Autodesk Fusion 360 part; units mm, degrees
sketch "Sketch1" plane through (0, 0, 0) normal (0, 1, 0) x (1, 0, 0)
  arc A0 (-2, -13.1375) -> (2, -13.1375) centre (0, -11.25) ccw
  line L0 (-2, -13.1375) -> (-2, -9.3625)
  arc A1 (2, -9.3625) -> (-2, -9.3625) centre (0, -11.25) ccw
  line L1 (2, -9.3625) -> (2, -13.1375)
  line L2 (-2.5, -13.3267) -> (-2.5, -9.1733)
  arc A2 (2.5, -9.1733) -> (-2.5, -9.1733) centre (0, -11.25) ccw
  line L3 (2.5, -9.1733) -> (2.5, -13.3267)
  arc A3 (-2.5, -13.3267) -> (2.5, -13.3267) centre (0, -11.25) ccw
  arc A4 (-6, -14.3423) -> (6, -14.3423) centre (0, -11.25) ccw
  line L4 (6, -8.1577) -> (6, -14.3423)
  arc A5 (6, -8.1577) -> (-6, -8.1577) centre (0, -11.25) ccw
  line L5 (-6, -14.3423) -> (-6, -8.1577)
  circle A6 centre (10, -11.25) radius 2.5
  line L6 (2.5219, -17.5112) -> (11.06, -13.5142)
  line L7 (3.1933, -5.3031) -> (11.06, -8.9858)
  line L8 (1.5, -9.5729) -> (1.5, -12.9271)
  arc A7 (-1.5, -12.9271) -> (1.5, -12.9271) centre (0, -11.25) ccw
  line L9 (-1.5, -12.9271) -> (-1.5, -9.5729)
  arc A8 (1.5, -9.5729) -> (-1.5, -9.5729) centre (0, -11.25) ccw
  circle A9 centre (0, -11.25) radius 6.75
  dimension "d1" = 0.5
  dimension "d2" = -4
  dimension "d3" = 5
  dimension "d4" = 10
  dimension "d7" = 0.5
  dimension "d10" = 13.5
extrude "Extrude1" add sketch "Sketch1" along normal blind 5 contours A4 L4 A5 L5 L6 A9 | L5 A9 | A4 A5 A6 L6 L7 A9 | L4 A9 | A6
extrude "Extrude2" add sketch "Sketch1" along normal blind 1.5 contours A0 L0 A1 L1 | L2 A2 L3 A3
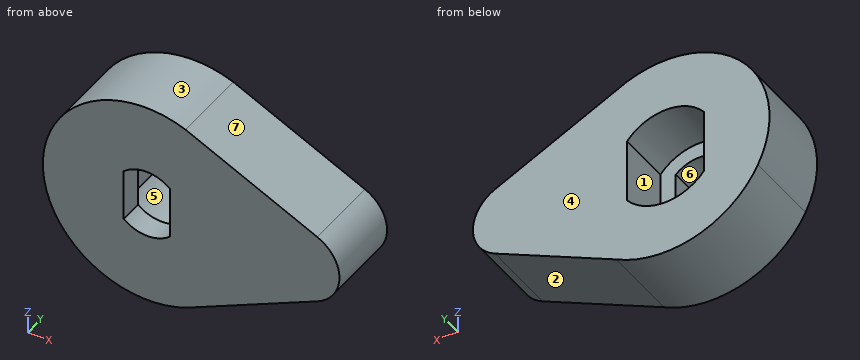
Geometry: final body of the model. Coordinates: model frame, mm. Face numbers are marked on the shaded views. A direction names the side the tool comes from. Round coordinates to 2 decimals unless told otherwise and drop trailing zeros. Write each loop counter-clockwise with the first axis right and the second up, starting at its lowest first coordinate (ties: lowest second). Pieces come first, ordered by that corner, then holes.
Item 1: Set-up query: the marked faces 5, 6 and 7. Return all of +Z, -Z, +X, -X, +Y, -Y with unobstructed straight access to the full face (end or side cutting, diameter ignored); none if empty.
Item 2: Section query B-B (z = 11.75). Return loops of the section in (x, y), plus the area to 3 significant figures.
Item 3: Material intervals for L1, parallel to X at y = 4.1, z = 9.5; L2, parallel to X at y = 0.35, z = 9.25; L3, parallel to Z at x = 0.75, y = 2.65, sorted ascending.
Item 4: Pin query (flat end, axial travel): P1, Ø1.5, axis at x = -1, z = 9, coming from the +Y side; P2, Ø0.8, axis at y = 1, z = 10.5, coming from the -X side; P3, Ø1.5, axis at x = 8.5, y = 3.5, coming from the -Z side. Return the tip coordinate at first contact, or that it passes through.
Item 5: Section query A-A (y = 0.95). Return loops of the section in (x, z), plus the area to 3 significant figures.
Item 6: Section query C-C (x = 1). Return loops of the section in (y, z).
Item 7: Mould query, pull axis X, two halves, no side actions, for the marked faces 1, 2, 3 and 4. Classes: +X half, -X half, draft (parallel to the pull), parting line (faces both ways), or undercut.
Item 8: Section query D-D (y = 1.8). Return loops of the section in (x, z).
Completed:
1. face 5: +Y
1. face 6: +Y, -Y
1. face 7: +Z, +X, +Y, -Y
2. outline: (-6.73, 0) - (-1.5, 0) - (-1.5, 1.5) - (-2.5, 1.5) - (-2.5, 5) - (-6.73, 5) - close; (1.5, 0) - (12.45, 0) - (12.45, 5) - (2.5, 5) - (2.5, 1.5) - (1.5, 1.5) - close
2. area: 73.9 mm2
3. L1: x = -6.52 to -2.5, 2.5 to 11.79
3. L2: x = -6.45 to -1.03, 1.03 to 11.5
3. L3: z = 4.54 to 8.09, 14.41 to 17.96
4. P1: stops at y = 1.5
4. P2: stops at x = -6.74
4. P3: stops at z = 7.44
5. outline: (2.52, 17.51) arc R6.75 ccw (long way) to (3.19, 5.3) - (11.06, 8.99) arc R2.5 ccw to (11.06, 13.51) - close; hole (-1.5, 9.57) arc R2.25 ccw to (1.5, 9.57) - (1.5, 12.93) arc R2.25 ccw to (-1.5, 12.93) - close
5. area: 170 mm2
6. outline: (0, 4.57) - (5, 4.57) - (5, 8.16) - (1.5, 8.16) - (1.5, 9.23) - (0, 9.23) - close; (0, 13.27) - (1.5, 13.27) - (1.5, 14.34) - (5, 14.34) - (5, 17.93) - (0, 17.93) - close
7. face 1: undercut
7. face 2: +X half
7. face 3: parting line
7. face 4: draft
8. outline: (2.52, 17.51) arc R6.75 ccw (long way) to (3.19, 5.3) - (11.06, 8.99) arc R2.5 ccw to (11.06, 13.51) - close; hole (-2.5, 9.17) arc R3.25 ccw to (2.5, 9.17) - (2.5, 13.33) arc R3.25 ccw to (-2.5, 13.33) - close
